Autodesk Inventor part; units mm, degrees
ref_plane "YZ Plane" through (0, 0, 0) normal (1, 0, 0) x (0, 1, 0)
ref_plane "XZ Plane" through (0, 0, 0) normal (0, 1, 0) x (-1, 0, 0)
ref_plane "XY Plane" through (0, 0, 0) normal (0, 0, 1) x (1, 0, 0)
sketch "Эскиз1" plane through (0, 0, 0) normal (0, 1, 0) x (-1, 0, 0)
  circle A0 centre (0, 0) radius 2.5
  dimension "d0" = 5
extrude "Выдавливание1" add sketch "Эскиз1" along normal blind 35
sketch "Эскиз2" plane through (0, 35, 0) normal (0, 1, 0) x (1, 0, 0)
  circle A0 centre (0, 0) radius 2.5
  line L0 (2.5, 0) -> (1.25, -2.1651)
  line L1 (1.25, -2.1651) -> (-1.25, -2.1651)
  line L2 (-1.25, -2.1651) -> (-2.5, 0)
  line L3 (-2.5, 0) -> (-1.25, 2.1651)
  line L4 (-1.25, 2.1651) -> (1.25, 2.1651)
  line L5 (1.25, 2.1651) -> (2.5, 0)
  point P0 (1.25, 2.1651)
  point P1 (1.25, 2.1651)
  point P2 (-2.5, 0)
  point P3 (-2.5, 0)
  point P4 (-1.25, -2.1651)
  point P5 (-1.25, -2.1651)
extrude "Выдавливание2" cut sketch "Эскиз2" against normal through all contours L5 A0 | A0 L0 | L4 A0 | A0 L1 | L3 A0 | A0 L2
sketch "Эскиз3" plane through (0, 0, 0) normal (0, -1, 0) x (1, 0, 0)
  circle A0 centre (0, 0) radius 1.5
  dimension "d5" = 3
extrude "Выдавливание3" cut sketch "Эскиз3" against normal through all
properties part number "Stoics"
Part model, mm, in its own coordinate system. Round coordinates to 2 decimals unless told otherwise and drop trailing zeros. Write each loop counter-clockwise with the first axis right and the second up, starting at its lowest first coordinate (ties: lowest second). Pieces come first, ordered by that corner, then holes. Notation, with made-up numbers: M 72.25,75.5 L 117.25,75.5 A16 cw 117.25,83.5 Z; hole C 0.5,5.5 d1. An arc over 180 degrees is marked long. One line per question, with ' | ' between items.
(1) Saw through at B-B on y = 23. Write the cut outline in (x, z), then the cut area to 3 significant figures.
Answer key:
outline: M -2.5,0 L -1.25,-2.17 L 1.25,-2.17 L 2.5,0 L 1.25,2.17 L -1.25,2.17 Z; hole C 0,0 d3 | area: 9.17 mm^2
(2) Saw through at C-C on z = 1. Write the cut outline in (x, y).
Answer key:
outline: M -1.92,0 L -1.12,0 L -1.12,35 L -1.92,35 Z; M 1.12,0 L 1.92,0 L 1.92,35 L 1.12,35 Z
(3) Pin check, flat tip, straight feed: pin 1 (2.5 mm diameter, centred on x = 0, z = 0, fed in from -Y). Stop position of the tip, or through.
Answer key:
pin 1: passes through
(4) Probe line 1 along Z through (x, y) = (0, 28.5); line 2 along X through (y, z) = (2.5, 0.45); line 3 along X through (y, z) = (4, 1.25). List the from-to ranges inside material, lowest first.
Answer key:
line 1: z = -2.17 to -1.5, 1.5 to 2.17 | line 2: x = -2.24 to -1.43, 1.43 to 2.24 | line 3: x = -1.78 to -0.83, 0.83 to 1.78
(5) Saw through at A-A on x = -0.9. Write the cut outline in (y, z), then the cut area to 3 significant figures.
Answer key:
outline: M 0,-2.17 L 35,-2.17 L 35,-1.2 L 0,-1.2 Z; M 0,1.2 L 35,1.2 L 35,2.17 L 0,2.17 Z | area: 67.6 mm^2
